from build123d import *

# Parameters (mm, degrees)
SKETCH_1_R          = 12.75
EXTRUDE_1_DEPTH     = 0.2
SKETCH_2_R          = 6.2
EXTRUDE_2_DEPTH     = 6
SKETCH_3_R          = 3.95
CUT_EXTRUDE_1_DEPTH = 20.067380523
CHAMFER_1_SIZE      = 0.5


with BuildPart() as part:
    # Эскиз1 → Бобышка-Вытянуть1 (new body)
    with BuildSketch(Plane(origin=(0, 0, 0), x_dir=(1, 0, 0), z_dir=(0, 1, 0))):
        with Locations(Location((0, 0, 0), (0, 0, 270))):
            Circle(SKETCH_1_R)
    extrude(amount=EXTRUDE_1_DEPTH)

    # Эскиз2 → Бобышка-Вытянуть2 (add)
    with BuildSketch(Plane(origin=(0, 0.2, 0), x_dir=(1, 0, 0), z_dir=(0, 1, 0))):
        with Locations(Location((0, 0, 0), (0, 0, 90))):
            Circle(SKETCH_2_R)
    extrude(amount=EXTRUDE_2_DEPTH)

    # Эскиз3 → Вырез-Вытянуть1 (cut, through all)
    with BuildSketch(Plane(origin=(0, 6.2, 0), x_dir=(1, 0, 0), z_dir=(0, 1, 0))):
        with Locations(Location((0, 0, 0), (0, 0, 270))):
            Circle(SKETCH_3_R)
    extrude(amount=-CUT_EXTRUDE_1_DEPTH, mode=Mode.SUBTRACT)

    # Фаска1
    chamfer_1_edges = [part.edges().sort_by_distance(p)[0] for p in [
        (0, 0, -3.95),
        (0, 6.2, -3.95),
        (0, 0.2, 6.2),
        (0, 6.2, 6.2),
    ]]
    chamfer(chamfer_1_edges, length=CHAMFER_1_SIZE)


solid = part.part
Could you check a few things on this model? Use its own coordinates, in mm. A direction names the side the tool comes from. Give positions to 0.01 mm unless a question says otherwise; leave off trailing zeros. Write each loop counter-clockwise with the first axis right and the second up, starting at its lowest first coordinate (ties: lowest second). Pieces come first, ordered by that corner, then holes. Notation, with made-up numbers: (78, 62) - (117, 62) arc R13 cw to (117, 73) - close; hole circle Ø8 at (-12.5, -20.5). An arc over 180 degrees is marked (long way). Use CSV: the item, a comma, the result in double quotes. Start each with the question number.
Item 1: For faces 1 (the face through (5, 6.2, 0)), 2 (the face through (-5, 0.2, 5)), which set-ups out of +Z, -Z, +X, -X, +Y, -Y let a thin tool reach every point of the face, with its end or its side?
Item 2: If we mould it in two halves opening along Z, with no side actions, what happens to faces 3 (the face through (0, 0, 5)), 4 (the face through (-1.9, 3.2, -5.9)), 5 (the face through (2.67, 3.14, -2.91))? For each: pulls with the +Z half, pulls with the -Z half, needs draft (parallel to the pull), parting line crosses it, or undercut.
Item 3: I want a section at A-A, the plane z = 0. Please give me the cut outline in (x, y).
Item 4: If I drill on line 1 along X through (y, z) = (2.9, 0); line 2 along Y through (x, z) = (1.25, -11.5); line 3 along X through (y, z) = (4, -1.25), over which ranges is the centre line in solid material (lowest first)?
Item 5: I want a section at C-C, the plane y = 4. Please give me the cut outline in (x, z), then the cut area to 3 significant figures.
Item 6: I'm going to push flat-ended pins straight in: pin 1 (1 mm diameter, centred on y = 4, z = -2, fed in from +X); pin 2 (2 mm diameter, centred on x = -0.5, y = 2.5, fed in from +Z); pin 3 (2 mm diameter, centred on x = -2.5, y = 2, fed in from +Z). Where does each tip first touch, or does it pass through?
Item 7: I want a section at D-D, the plane x = 9.75. Please give me the cut outline in (y, z), then the cut area to 3 significant figures.
Item 8: I want a section at B-B, the plane x = 0. Please give me the cut outline in (y, z).
Findings:
1,face 1,"+Z, -Z, +X, -X, +Y"
1,face 2,"+Y"
2,face 3,"needs draft"
2,face 4,"parting line crosses it"
2,face 5,"undercut"
3,outline,"(-12.75, 0) - (-4.45, 0) - (-3.95, 0.5) - (-3.95, 5.7) - (-4.45, 6.2) - (-5.7, 6.2) - (-6.2, 5.7) - (-6.2, 0.7) - (-6.7, 0.2) - (-12.75, 0.2) - close; (3.95, 0.5) - (4.45, 0) - (12.75, 0) - (12.75, 0.2) - (6.7, 0.2) - (6.2, 0.7) - (6.2, 5.7) - (5.7, 6.2) - (4.45, 6.2) - (3.95, 5.7) - close"
4,line 1,"x = -6.2 to -3.95, 3.95 to 6.2"
4,line 2,"y = 0 to 0.2"
4,line 3,"x = -6.07 to -3.75, 3.75 to 6.07"
5,outline,"circle Ø12.4 at (0, 0); hole circle Ø7.9 at (0, 0)"
5,area,"71.7 mm2"
6,pin 1,"stops at x = 6.02"
6,pin 2,"stops at z = 6.2"
6,pin 3,"stops at z = 6.02"
7,outline,"(0, -8.22) - (0.2, -8.22) - (0.2, 8.22) - (0, 8.22) - close"
7,area,"3.29 mm2"
8,outline,"(0, -12.75) - (0.2, -12.75) - (0.2, -6.7) - (0.7, -6.2) - (5.7, -6.2) - (6.2, -5.7) - (6.2, -4.45) - (5.7, -3.95) - (0.5, -3.95) - (0, -4.45) - close; (0, 4.45) - (0.5, 3.95) - (5.7, 3.95) - (6.2, 4.45) - (6.2, 5.7) - (5.7, 6.2) - (0.7, 6.2) - (0.2, 6.7) - (0.2, 12.75) - (0, 12.75) - close"
